Model file for the job. Use its own axes, mm. Round coordinates to 2 decimals unless told otherwise and drop trailing zeros. Write each loop counter-clockwise with the first axis right and the second up, starting at its lowest first coordinate (ties: lowest second). Pieces come first, ordered by that corner, then holes. Notation, with made-up numbers: (29, 71) - (83, 71) arc R30 ccw to (83, 98) - close; hole circle Ø8 at (-25.75, 12). An arc over 180 degrees is marked (long way). One line per item, written item: value.
Autodesk Inventor part; units mm, degrees
ref_plane "YZ Plane" through (0, 0, 0) normal (1, 0, 0) x (0, 1, 0)
ref_plane "XZ Plane" through (0, 0, 0) normal (0, 1, 0) x (-1, 0, 0)
ref_plane "XY Plane" through (0, 0, 0) normal (0, 0, 1) x (1, 0, 0)
sketch "Esboço1" plane through (0, 0, 0) normal (0, 1, 0) x (-1, 0, 0)
  line L0 (0, 0) -> (35, 0)
  line L1 (35, 0) -> (35, -47)
  line L2 (35, -47) -> (0, -47)
  line L3 (0, -47) -> (0, 0)
  dimension "d0" = 35
  dimension "d1" = 47
extrude "Extrusão1" add sketch "Esboço1" along normal blind 2
fillet "Arredondamento1" radius 2 4 edges at (0, 1, 0) (0, 1, -47) (-35, 1, 0) (-35, 1, -47)
sketch "Esboço5" plane through (0, 2, 0) normal (0, 1, 0) x (1, 0, 0)
  circle A0 centre (-4.5, 42.5) radius 1.505
  line L0 (-2, 47) -> (-33, 47)
  line L1 (0, 2) -> (0, 45)
  circle A1 centre (-30.5, 42.5) radius 1.505
  circle A2 centre (-4.5, 4.5) radius 1.505
  circle A3 centre (-30.5, 4.5) radius 1.505
  point P0 (0, 0)
  dimension "d26" = 3.01
  dimension "d27" = 4.5
  dimension "d28" = 4.5
  dimension "d31" = 26
  dimension "d34" = 38
extrude "Extrusão4" cut sketch "Esboço5" against normal blind 4.5
equation "\"d37\" = d28"
properties part number "Tampa"
1. Wall check: probe 1 along Z at (x, y) = (-4.5, 0.6) (3 decimals); probe 2 along X at (y, z) = (0.75, -42.5) (3 decimals); probe 3 along X at (y, z) = (1.65, -3.5). Give the ranges that are in metal, low to high. Write a range as [from, to].
Report:
probe 1: [-47, -44.005], [-40.995, -6.005], [-2.995, 0]
probe 2: [-35, -32.005], [-28.995, -6.005], [-2.995, 0]
probe 3: [-35, -31.62], [-29.38, -5.62], [-3.38, 0]
2. Band-saw the part on C-C on z = -42.5. Write the cut outline in (x, y) (3 decimals), plus the area to 3 significant figures.
Report:
outline: (-35, 0) - (-32.005, 0) - (-32.005, 2) - (-35, 2) - close; (-28.995, 0) - (-6.005, 0) - (-6.005, 2) - (-28.995, 2) - close; (-2.995, 0) - (0, 0) - (0, 2) - (-2.995, 2) - close
area: 58.0 mm²
3. Band-saw the part on B-B on x = -4.5. Write the cut outline in (y, z) (3 decimals), plus the area to 3 significant figures.
Report:
outline: (0, -47) - (2, -47) - (2, -44.005) - (0, -44.005) - close; (0, -40.995) - (2, -40.995) - (2, -6.005) - (0, -6.005) - close; (0, -2.995) - (2, -2.995) - (2, 0) - (0, 0) - close
area: 82.0 mm²
4. Mould opens along Z. For faces 1 (the face through (-35, 1, -23)), 2 (the face through (-4.83, 1.01, -41.03)), 3 (the face through (-3.064, 1.014, -4.952)), 4 (the face through (-34.43, 1.01, -0.6)) say: released by +Z, released by -Z, zero draft, split by the parting line, or undercut.
Report:
face 1: zero draft
face 2: undercut
face 3: undercut
face 4: released by +Z
5. Band-saw the part on A-A on y = 1. Write the cut outline in (x, z) (3 decimals).
Report:
outline: (-35, -45) arc R2 ccw to (-33, -47) - (-2, -47) arc R2 ccw to (0, -45) - (0, -2) arc R2 ccw to (-2, 0) - (-33, 0) arc R2 ccw to (-35, -2) - close; hole circle Ø3.01 at (-30.5, -42.5); hole circle Ø3.01 at (-30.5, -4.5); hole circle Ø3.01 at (-4.5, -42.5); hole circle Ø3.01 at (-4.5, -4.5)
